Autodesk Fusion 360 part; units mm, degrees
sketch "Sketch1" plane through (0, 0, 0) normal (0, 0, 1) x (1, 0, 0)
  line L0 (15, 0) -> (65.0001, 0)
  line L1 (65.0001, 30) -> (15, 30)
  arc A0 (65.0001, 0) -> (65.0001, 30) centre (65, 15) ccw
  arc A1 (15, 30) -> (15, 0) centre (15, 15) ccw
  line L2 (0, 0) -> (0, 40.5539) construction
  line L3 (0, 0) -> (80, 0) construction
  dimension "d9" = 15
  dimension "d10" = 50
extrude "Extrude1" add sketch "Sketch1" along normal blind 3
sketch "Sketch2" plane through (0, 0, 3) normal (0, 0, 1) x (-1, 0, 0)
  arc A0 (-15, -30) -> (-15, 0) centre (-15, -15) ccw
  line L0 (-15, 0) -> (-65.0001, 0)
  arc A1 (-65.0001, 0) -> (-65.0001, -30) centre (-65, -15) ccw
  line L1 (-65.0001, -30) -> (-15, -30)
  arc A2 (-65.0001, -3) -> (-65, -27) centre (-65, -15) ccw
  line L2 (-65, -27) -> (-15, -27)
  arc A3 (-15, -27) -> (-15, -3) centre (-15, -15) ccw
  line L3 (-15, -3) -> (-65.0001, -3)
  line L4 (-65, -15) -> (-65.0001, 0) construction
  line L5 (-65.0001, 0) -> (-15.0001, 0.0002) construction
  line L6 (-15.0001, 0.0002) -> (-15, -15) construction
  line L7 (-15, -15) -> (-65, -15) construction
  arc A4 (-69.8903, -4.0417) -> (-60.0001, -3) centre (-65.0001, -3) ccw
  arc A5 (-45, -3) -> (-35, -3) centre (-40, -3.0001) ccw
  arc A6 (-20, -3) -> (-10.1097, -4.0417) centre (-15, -3) ccw
  arc A7 (-18.9998, 0.0002) -> (-19, 0) centre (-15, -3) ccw
  arc A8 (-20, -3) -> (-10.1097, -4.0417) centre (-15, -3) ccw
  arc A9 (-45, -3) -> (-35, -3) centre (-40, -3.0001) ccw
  arc A10 (-69.8903, -4.0417) -> (-60.0001, -3) centre (-65.0001, -3) ccw
  line L8 (-15.0001, -14.9998) -> (-15, -30) construction
  line L9 (-15, -30) -> (-15.9207, -30) construction
  line L10 (-15, -30) -> (-65, -30) construction
  arc A11 (-35, -27) -> (-45, -27) centre (-40, -27) ccw
  arc A12 (-10.1097, -25.9583) -> (-20, -27) centre (-15, -27) ccw
  arc A13 (-60, -27) -> (-69.8903, -25.9583) centre (-65, -27) ccw
  circle A14 centre (-15, -27) radius 1.5
  circle A15 centre (-40, -27) radius 1.5
  circle A16 centre (-65, -27) radius 1.5
  circle A17 centre (-15, -3) radius 1.5
  circle A18 centre (-40, -3) radius 1.5
  circle A19 centre (-65, -3) radius 1.5
  circle A20 centre (-40, -3) radius 2.5
  circle A21 centre (-65, -3) radius 2.5
  circle A22 centre (-65, -27) radius 2.5
  circle A23 centre (-40, -27) radius 2.5
  circle A24 centre (-15, -27) radius 2.5
  circle A25 centre (-15, -3) radius 2.5
  dimension "d13" = -3
  dimension "d44" = 10
  dimension "d47" = 10
  dimension "d48" = 10
  dimension "d51" = 10
  dimension "d52" = 10
  dimension "d53" = 10
  dimension "d55" = 10
  dimension "d56" = 10
  dimension "d57" = 10
  dimension "d60" = 3
  dimension "d61" = 3
  dimension "d62" = 3
  dimension "d63" = 3
  dimension "d64" = 3
  dimension "d65" = 3
  dimension "d66" = 1
  dimension "d67" = 1
  dimension "d68" = 1
  dimension "d69" = 1
  dimension "d70" = 1
  dimension "d71" = 1
extrude "Extrude2" add sketch "Sketch2" along normal blind 14 contours A0 L0 A1 L1 A2 L2 A3 L3 A7 A20 A21 A22 A23 A24 | A0 L0 A3 L3 A7 A25 | A3 L3 A17 A25 | L2 A3 A14 A24 | A3 L3 A17 | L3 A18 A20 | L2 A3 A14 | L3 A18 | L2 A15 A23 | A2 L3 A19 A21 | L2 A15 | A2 L3 A19 | A2 L2 A16 A22 | A2 L2 A16 picked at (-13.0721, -2.848) picked at (-13.0721, -27.152) picked at (-14.6506, -2.538) picked at (-42.1518, -2.8013) picked at (-14.6506, -27.462) picked at (-40.339, -2.2448) picked at (-42.1518, -27.1987) picked at (-66.9146, -2.7753) picked at (-39.7775, -27.9749) picked at (-65.3253, -2.5293) picked at (-66.9146, -27.2247) picked at (-65.3252, -27.4707)
sketch "Sketch3" plane through (0, 0, 0) normal (0, 0, -1) x (1, 0, 0)
  arc A0 (15, 0) -> (15, -30) centre (15, -15) ccw
  line L0 (15, -30) -> (65.0001, -30)
  arc A1 (65.0001, -30) -> (65.0001, 0) centre (65, -15) ccw
  line L1 (65.0001, 0) -> (15, 0)
  line L2 (65, -15) -> (65.0001, 0) construction
  line L3 (65, -15) -> (15, -15) construction
  line L4 (15, -15) -> (15, 0) construction
  line L5 (15, 0) -> (65.0001, 0) construction
  line L6 (15, 0) -> (15, -3) construction
  line L7 (18, -3) -> (18, 0) construction
  line L8 (18, 0) -> (12, 0) construction
  line L9 (12, 0) -> (12, -3) construction
  line L10 (12, -3) -> (12, 0) construction
  line L11 (15, 0) -> (18, 0) construction
  line L12 (18, 0) -> (18, -3) construction
  line L13 (12, -3) -> (12, 0)
  line L14 (12, 0) -> (18, 0)
  line L15 (18, 0) -> (18, -3)
  arc A2 (12, -3) -> (18, -3) centre (15, -3) ccw
  line L16 (40, -3) -> (43, -3) construction
  line L17 (43, 0) -> (37, 0) construction
  line L18 (37, 0) -> (43, 0)
  line L19 (43, 0) -> (43, -3)
  line L20 (37, -3) -> (37, 0)
  arc A3 (37, -2.998) -> (43, -3) centre (40, -3) ccw
  line L21 (65, -3) -> (68, -3) construction
  arc A4 (65.0066, 0) -> (64.9934, 0) centre (65, -3) ccw
  arc A5 (68, -27) -> (62, -27) centre (65, -27) ccw
  line L22 (62, -30) -> (62, -27)
  line L23 (68, -27) -> (68, -30)
  arc A6 (43, -27.002) -> (37, -27) centre (40, -27) ccw
  line L24 (43, -27) -> (43, -30)
  line L25 (37, -30) -> (37, -27)
  line L26 (18, -27) -> (18, -30)
  arc A7 (18, -27.0025) -> (12, -27) centre (15, -27) ccw
  line L27 (12, -30) -> (12, -27)
  line L28 (68, 0) -> (68, -3)
  arc A8 (62, -2.998) -> (68, -3) centre (65, -3) ccw
  line L29 (62, -3) -> (62, 0)
  line L30 (62, 0) -> (68, 0)
  dimension "d16" = 6
  dimension "d17" = 6
  dimension "d23" = 6
  dimension "d25" = 6
  dimension "d27" = 6
  dimension "d28" = 6
  dimension "d29" = 6
  dimension "d40" = 6
extrude "Extrude3" cut sketch "Sketch3" against normal blind 3 contours A0 L1 L13 L14 L15 A2
extrude "Extrude4" cut sketch "Sketch3" against normal blind 3 contours L1 L18 L19 L20 A3
extrude "Extrude5" cut sketch "Sketch3" against normal blind 3 contours L0 A6 L24 L25
extrude "Extrude6" cut sketch "Sketch3" against normal blind 3 contours A0 L0 L26 A7 L27
extrude "Extrude7" cut sketch "Sketch3" against normal blind 3 contours L0 A1 A5 L22 L23
extrude "Extrude8" cut sketch "Sketch3" against normal blind 3 contours A1 L1 A4 L28 A8 L29 L30
extrude "Extrude9" add sketch "Sketch2" along normal blind 1 contours A2 L3 A4 A10 A21 | A2 L3 A19 A21 | A2 L3 A19 picked at (-66.8477, -3.5405) picked at (-65.3313, -3.4756)
extrude "Extrude10" add sketch "Sketch2" along normal blind 1 contours A3 L3 A6 A7 A8 A25 | A3 L3 A17 A25 | L3 A5 A9 A20 | A3 L3 A17 | L3 A18 A20 | L3 A18 picked at (-13.1523, -3.5405) picked at (-14.6688, -3.4756) picked at (-42.1574, -3.1242) picked at (-40.3832, -3.562)
extrude "Extrude11" add sketch "Sketch2" along normal blind 1 contours L2 A3 A12 A24 | L2 A3 A14 A24 | L2 A3 A14 | L2 A11 A23 | L2 A15 A23 | L2 A15 | A2 L2 A13 A22 | A2 L2 A16 A22 | A2 L2 A16 picked at (-13.1523, -26.4595) picked at (-14.6688, -26.5244) picked at (-42.1574, -26.8758) picked at (-39.6335, -26.6599) picked at (-66.8477, -26.4595) picked at (-65.3313, -26.5244)
extrude "Extrude12" add sketch "Sketch2" along normal blind 14 contours A3 L3 A17 A25 | A3 L3 A17 A25 | A3 L3 A17 | A3 L3 A17
extrude "Extrude13" cut sketch "Sketch2" along normal blind 15 contours A3 L3 A17 | A3 L3 A17
extrude "Extrude14" add sketch "Sketch2" along normal blind 14 contours A3 L3 A17 A25 | A3 L3 A17 A25 | L2 A3 A14 A24 | L2 A3 A14 A24 | A3 L3 A17 | A3 L3 A17 | L3 A18 A20 | L3 A18 A20 | L2 A3 A14 | L2 A3 A14 | L3 A18 | L3 A18 | L2 A15 A23 | L2 A15 A23 | A2 L3 A19 A21 | A2 L3 A19 A21 | L2 A15 | L2 A15 | A2 L3 A19 | A2 L3 A19
extrude "Extrude15" add sketch "Sketch2" along normal blind 14 contours A2 L2 A16 A22 | A2 L2 A16 A22 | A2 L2 A16 | A2 L2 A16
extrude "Extrude16" cut sketch "Sketch2" along normal blind 15 contours A3 L3 A17 | A3 L3 A17 | L2 A3 A14 | L2 A3 A14 | L3 A18 | L3 A18 | L2 A15 | L2 A15 | A2 L3 A19 | A2 L3 A19 | A2 L2 A16 | A2 L2 A16
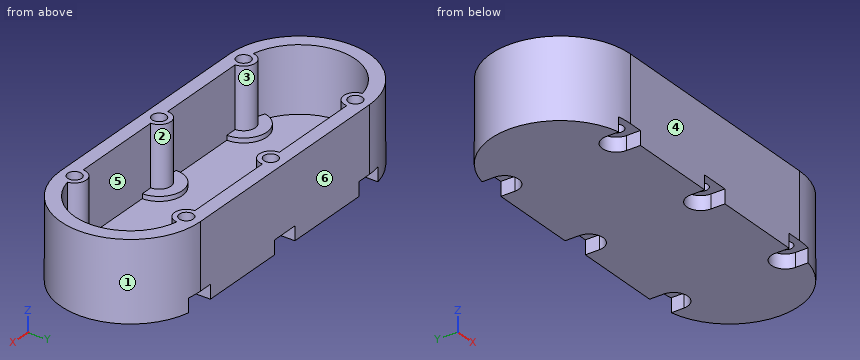
Source: CAD feature listing. Evaluate the final solid. Frame: model axes, mm. Face numbers are marked on the shaded views. A direction names the side the tool comes from. Give positions to 0.01 mm unless a question says otherwise; leave off trailing zeros. Write each loop counter-clockwise with the first axis right and the second up, starting at its lowest first coordinate (ties: lowest second). Pieces come first, ordered by that corner, then holes.
1. Access query for the marked faces 5 and 6. Directions: +Z, -Z, +X, -X, +Y, -Y. A direction counts if a zero-diameter tool reaches every point of the face in a straight line with its end or side. Return the directions, or none.
2. Section query C-C (z = 11.5). Return the cut outline in (x, y).
3. Section query A-A (z = 1.5). Return the cut outline in (x, y).
4. Section query B-B (x = 40). Return the cut outline in (y, z).
5. Material intervals for line 1 along Y through (x, z) = (40, 6.75); line 2 along Y through (x, z) = (25.5, 3.75); line 3 along X through (y, z) = (5, 12.25), sorted ascending.
6. Pull-direction query (Y, two-part tool) for the marked faces 1, 2, 3 and 4; classes: +Y half, -Y half, draft (parallel to the pull), parting line (faces both ways), or undercut.
7. Section query D-D (y = 15). Return the cut outline in (x, z).
8. First-contact query: pin 1 (5 mm diameter, centred on x = 15, y = 27, fed in from -Z); pin 2 (0.9 mm diameter, centred on y = 29, z = 1.5, fed in from -X); pin 3 (5 mm diameter, centred on x = 58.5, y = 7.5, fed in from +Z); pin 4 (1 mm diameter, centred on x = 49.5, z = 5.5, fed in from -Y). Flat tips, straight axial feed; report the tip coordinate or a pass-through.
Output values:
1. face 5: +Z
1. face 6: +Z, -Z, +X, -X, +Y
2. outline: (15, 0) - (65, 0) arc R15 ccw to (65, 30) - (15, 30) arc R15 ccw to start; hole (12.51, 3.26) arc R2.5 cw to (17.5, 3) - (37.5, 3) arc R2.5 cw to (42.5, 3) - (62.5, 3) arc R2.5 cw to (67.49, 3.26) arc R12 ccw to (67.49, 26.74) arc R2.5 cw to (62.5, 27) - (42.5, 27) arc R2.5 cw to (37.5, 27) - (17.5, 27) arc R2.5 cw to (12.51, 26.74) arc R12 ccw to start; hole circle Ø3 at (15, 3); hole circle Ø3 at (15, 27); hole circle Ø3 at (40, 3); hole circle Ø3 at (40, 27); hole circle Ø3 at (65, 3); hole circle Ø3 at (65, 27)
3. outline: (12, 0.3) - (12, 3) arc R3 cw to (18, 3) - (18, 0) - (37, 0) - (37, 3) arc R3 cw to (43, 3) - (43, 0) - (62, 0) - (62, 3) arc R3 cw to (68, 3) - (68, 0.3) arc R15 ccw to (68, 29.7) - (68, 27) arc R3 cw to (62, 27) - (62, 30) - (43, 30) - (43, 27) arc R3 cw to (37, 27) - (37, 30) - (18, 30) - (18, 27) arc R3 cw to (12, 27) - (12, 29.7) arc R15 ccw to start
4. outline: (0, 3) - (1.5, 3) - (1.5, 17) - (0, 17) - close; (4.5, 3) - (6, 3) - (6, 0) - (24, 0) - (24, 3) - (25.5, 3) - (25.5, 17) - (24.5, 17) - (24.5, 4) - (22, 4) - (22, 3) - (8, 3) - (8, 4) - (5.5, 4) - (5.5, 17) - (4.5, 17) - close; (28.5, 3) - (30, 3) - (30, 17) - (28.5, 17) - close
5. line 1: y = 0 to 1.5, 4.5 to 5.5, 24.5 to 25.5, 28.5 to 30
5. line 2: y = 0 to 3, 27 to 30
5. line 3: x = 3.82 to 8.37, 13.5 to 16.5, 38.5 to 41.5, 63.5 to 66.5, 71.63 to 76.18
6. face 1: parting line
6. face 2: undercut
6. face 3: undercut
6. face 4: -Y half
7. outline: (0, 0) - (80, 0) - (80, 17) - (77, 17) - (77, 3) - (3, 3) - (3, 17) - (0, 17) - close
8. pin 1: stops at z = 3
8. pin 2: stops at x = 8.57
8. pin 3: stops at z = 3
8. pin 4: stops at y = 0
